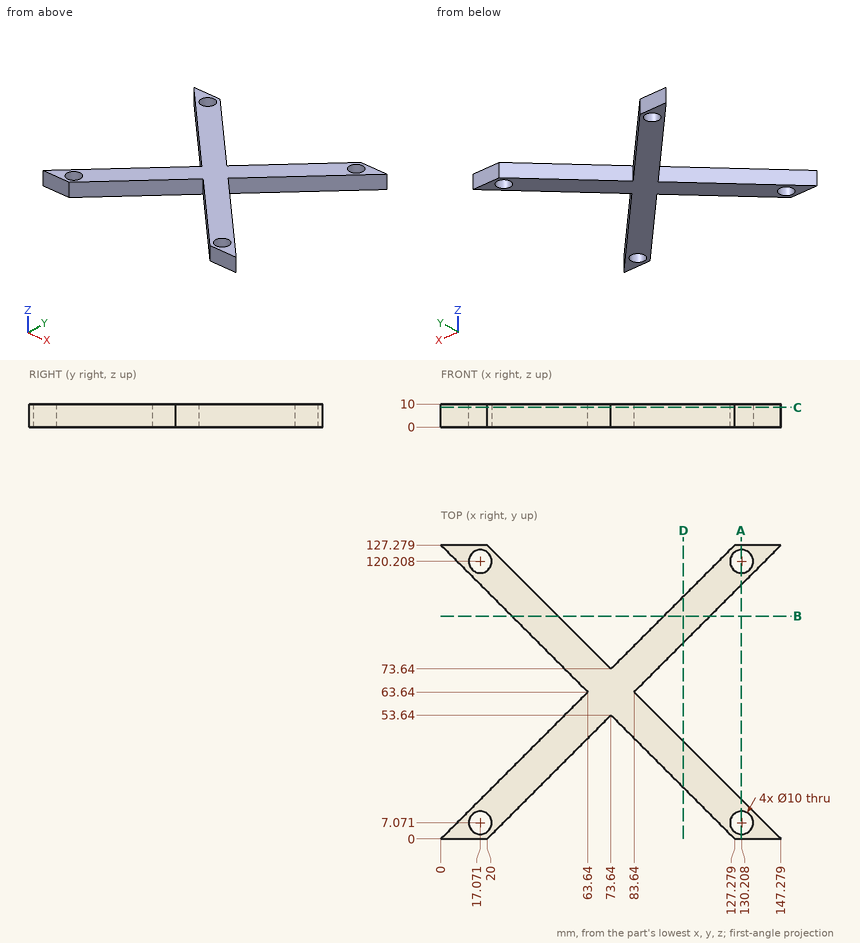
Answer from the drawing. Dimensions are ordinates in mm from the lowest x, y and z of the part. Give positions to 0.01 mm unless a question says otherwise; leave off trailing zeros. Write each loop counter-clockwise with the first axis right and the second up, starting at its lowest first coordinate (ties: lowest second). Pieces come first, ordered by that corner, then holes. Notation, with made-up numbers: (19.25, 88) - (70.25, 88) arc R9 ccw to (70.25, 105) - close; hole circle Ø9 at (-11.5, 81.25). An arc over 180 degrees is marked (long way). Answer in a Markdown table with one row per item. Add a question column.
Item 1: Flat-ended cylindrical pins translate along their axes: P1, Ø2, axis at x = 23, z = 7, coming from the -Y side; P2, Ø5, axis at y = 23.5, z = 3.5, coming from the +X side; P3, Ø2, axis at y = 63, z = 9, coming from the +X side; P4, Ø13, axis at x = 130.21, y = 7.07, coming from the -Z side. Find the tip coordinate at first contact, or state that the pin passes through.
Item 2: Section A-A, the plane x = 130 is taken. Write down the section's boundary in (y, z) (1 decimal), and give its area (3 significant figures).
Item 3: Section B-B, the plane y = 96.5 is taken. Write down the section's boundary in (x, z).
Item 4: Section D-D, the plane x = 105 is taken. Write down the section's boundary in (y, z).
Item 5: Find the intervals of material crossed by L1, parallel to X at y = 118, z = 2.25 (1 decimal); L2, parallel to Y at x = 101, z = 2.5; L3, parallel to X at y = 18, z = 3.5, in increasing order.
Item 6: Section C-C, the plane z = 8.5 is taken. Write down the section's boundary in (x, y).
Recorded:
| question | item | result |
|---|---|---|
| 1 | P1 | stops at y = 2 |
| 1 | P2 | stops at x = 126.28 |
| 1 | P3 | stops at x = 85.28 |
| 1 | P4 | stops at z = 0 |
| 2 | outline | (0, 0) - (2.1, 0) - (2.1, 10) - (0, 10) - close; (12.1, 0) - (17.3, 0) - (17.3, 10) - (12.1, 10) - close; (110, 0) - (115.2, 0) - (115.2, 10) - (110, 10) - close; (125.2, 0) - (127.3, 0) - (127.3, 10) - (125.2, 10) - close |
| 2 | area | 146 mm2 |
| 3 | outline | (30.78, 0) - (50.78, 0) - (50.78, 10) - (30.78, 10) - close; (96.5, 0) - (116.5, 0) - (116.5, 10) - (96.5, 10) - close |
| 4 | outline | (22.28, 0) - (42.28, 0) - (42.28, 10) - (22.28, 10) - close; (85, 0) - (105, 0) - (105, 10) - (85, 10) - close |
| 5 | L1 | x = 9.3 to 12.6, 21.6 to 29.3, 118 to 125.7, 134.7 to 138 |
| 5 | L2 | y = 26.28 to 46.28, 81 to 101 |
| 5 | L3 | x = 18 to 38, 109.28 to 129.28 |
| 6 | outline | (0, 0) - (20, 0) - (73.64, 53.64) - (127.28, 0) - (147.28, 0) - (83.64, 63.64) - (147.28, 127.28) - (127.28, 127.28) - (73.64, 73.64) - (20, 127.28) - (0, 127.28) - (63.64, 63.64) - close; hole circle Ø10 at (17.07, 7.07); hole circle Ø10 at (17.07, 120.21); hole circle Ø10 at (130.21, 7.07); hole circle Ø10 at (130.21, 120.21) |
